```python
from build123d import *

# Parameters (mm, degrees)
ESQUISSE1_R          = 11.3
BASE_EXTRUSION_DEPTH = 3
CHANFREIN1_SIZE      = 1


with BuildPart() as part:
    # Esquisse1 → Base-Extrusion (new, symmetric)
    with BuildSketch(Plane(origin=(0, 0, 0), x_dir=(1, 0, 0), z_dir=(0, 1, 0))):
        Polygon((8.631386524, 14.95), (17.262773049, 0), (8.631386524, -14.95), (-8.631386524, -14.95), (-17.262773049, 0), (-8.631386524, 14.95), align=None)
        with Locations(Location((0, 0, 0), (0, 0, 90))):
            Circle(ESQUISSE1_R, mode=Mode.SUBTRACT)
    extrude(amount=BASE_EXTRUSION_DEPTH, both=True)

    # Chanfrein1
    chanfrein1_edges = [part.edges().sort_by_distance(p)[0] for p in [
        (0, 3, 11.3),
        (0, -3, 11.3),
    ]]
    chamfer(chanfrein1_edges, length=CHANFREIN1_SIZE)

    # Esquisse2 → Enlèvement de matière-Révolution3 (revolve, cut)
    with BuildSketch(Plane.XY):
        Polygon((15.396747645, 3), (17.262773049, 2.5), (17.262773049, 3), align=None)
        Polygon((17.262773049, -3), (15.396747645, -3), (17.262773049, -2.5), align=None)
    revolve(axis=Axis((0, 0, 0), (0, -1, 0)), mode=Mode.SUBTRACT)


solid = part.part
```
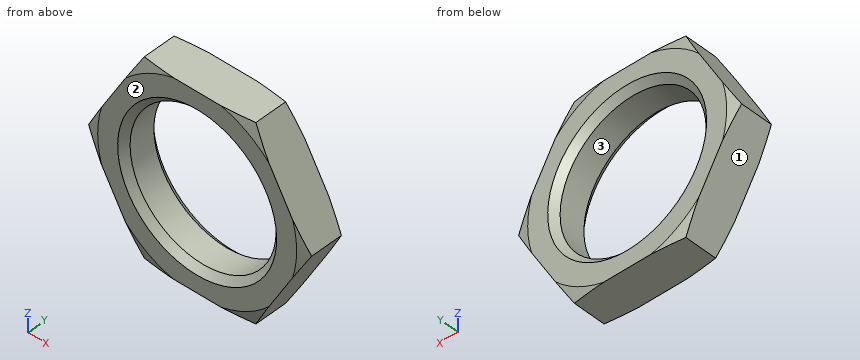
Design review of the part built by this model. Coordinates are the model's own, in mm. Face numbers are marked on the shaded views. Coordinates: 2 decimals unless noted, no trailing zeros. Write each loop counter-clockwise with the first axis right and the second up, starting at its lowest first coordinate (ties: lowest second). Pieces come first, ordered by that corner, then holes.
1) Add section B-B (x = 0). Write out the cut boundary in (y, z).
2) Add section A-A (y = 1). Write out the cut boundary in (x, z).
3) Insertion check: pin 1 (1.5 mm diameter, centred on x = -6.5, z = -6.5, fed in from -Y); pin 2 (10 mm diameter, centred on x = -13.5, z = -11, fed in from +Y); pin 3 (3 mm diameter, centred on y = 0, z = -4, fed in from -X). Each pin has a flat end and moves straight along its axis. Give the tip position at first contact, or say it passes through.
4) Mouldability with a two-part tool opening along X and no side actions: class the marked faces 1, 2 and 3 as +X half, -X half, draft (parallel to the pull), parting line (faces both ways), or undercut.
5) Add section C-C (x = 14). Write out the cut boundary in (y, z).
6) To check wall thickness, follow L1, parallel to Z at x = -5, y = 2.5; L2, parallel to X at y = -1.25, z = -2.5; L3, parallel to X at y = -0.25, z = 5.75. State the ranges of each line that lie inside material, in increasing order.
Check result:
1. outline: (-3, -14.95) - (3, -14.95) - (3, -12.3) - (2, -11.3) - (-2, -11.3) - (-3, -12.3) - close; (-3, 12.3) - (-2, 11.3) - (2, 11.3) - (3, 12.3) - (3, 14.95) - (-3, 14.95) - close
2. outline: (-17.26, 0) - (-8.63, -14.95) - (8.63, -14.95) - (17.26, 0) - (8.63, 14.95) - (-8.63, 14.95) - close; hole circle Ø22.6 at (0, 0)
3. pin 1: passes through
3. pin 2: stops at y = 3
3. pin 3: stops at x = -15.82
4. face 1: -X half
4. face 2: draft
4. face 3: undercut
5. outline: (-3, -5.65) - (3, -5.65) - (3, 5.65) - (-3, 5.65) - close
6. L1: z = -14.95 to -10.69, 10.69 to 14.95
6. L2: x = -15.82 to -11.02, 11.02 to 15.82
6. L3: x = -13.94 to -9.73, 9.73 to 13.94
